Geometry: see drawing. Coordinates: mm, zero at the bounding-box minimum. Coordinates: 2 decimals unless noted, no trailing zeros. Loops run counter-clockwise (first coordinate to the right, second up) from the corner with the lowest first, then second, coordinate; pieces in that order, holes last. Notation, with made-up numbers: (75, 55.5) - (120, 55.5) arc R25 ccw to (120, 70.5) - close; hole circle Ø8 at (-20.75, -26). An arc over 180 degrees is marked (long way). Use one line per item in the form item = value.
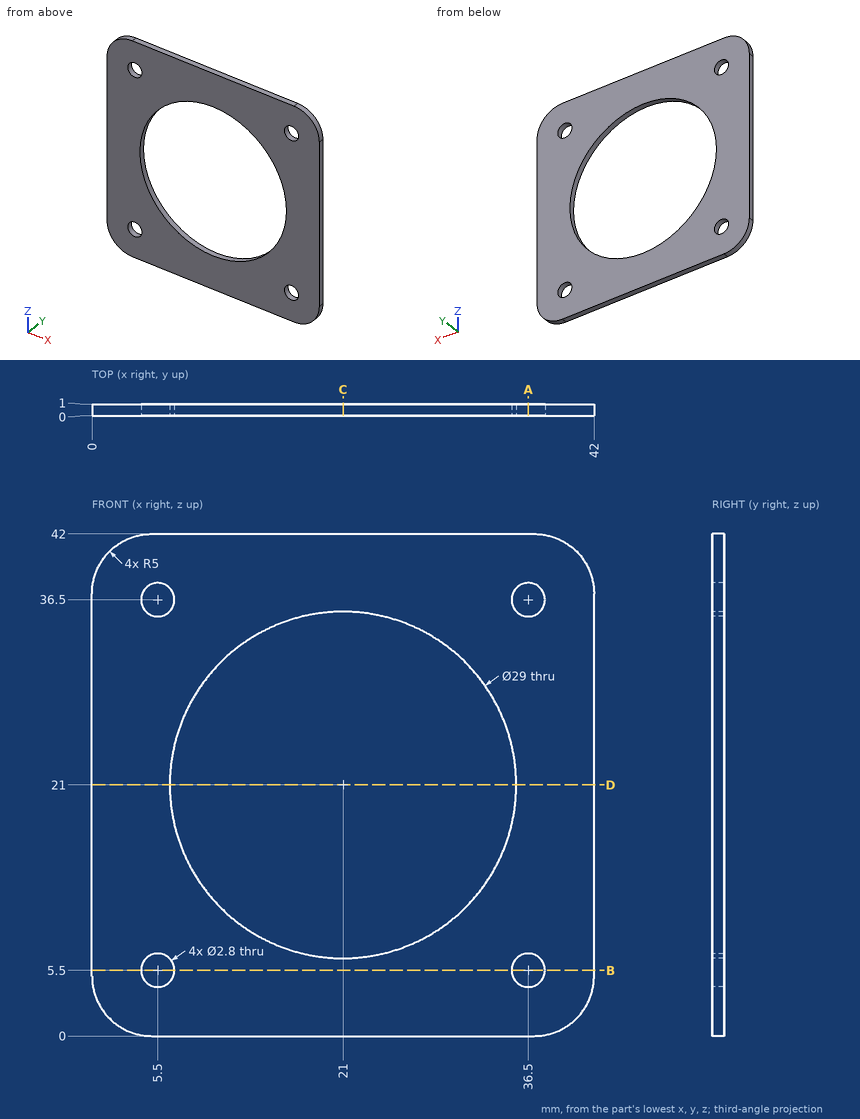
Q1. Cut plane B-B, the plane z = 5.5. Return loops of the section in (x, y).
Check values:
outline = (0, 0) - (4.1, 0) - (4.1, 1) - (0, 1) - close; (6.9, 0) - (35.1, 0) - (35.1, 1) - (6.9, 1) - close; (37.9, 0) - (42, 0) - (42, 1) - (37.9, 1) - close
Q2. First-contact query: P1, Ø3.5, axis at x = 5.5, z = 5.5, coming from the +Y side. Flat tip, straight axial feed; report the tip coordinate or a pass-through.
Check values:
P1 = 1
Q3. Cut plane A-A, the plane x = 36.5. Return loops of the section in (y, z), then the cut area to 3 significant figures.
Check values:
outline = (0, 0) - (1, 0) - (1, 4.1) - (0, 4.1) - close; (0, 6.9) - (1, 6.9) - (1, 35.1) - (0, 35.1) - close; (0, 37.9) - (1, 37.9) - (1, 42) - (0, 42) - close
area = 36.4 mm²
Q4. Cut plane D-D, the plane z = 21. Return loops of the section in (x, y), then the cut area to 3 significant figures.
Check values:
outline = (0, 0) - (6.5, 0) - (6.5, 1) - (0, 1) - close; (35.5, 0) - (42, 0) - (42, 1) - (35.5, 1) - close
area = 13.0 mm²
Q5. Ray query, line 1 along Z through (x, y) = (5.5, 0.6); line 2 along X through (y, z) = (0.15, 20.5). Return the intervals inside material, ascending. Write a range as [from, to].
Check values:
line_1 = [0, 4.1], [6.9, 35.1], [37.9, 42]
line_2 = [0, 6.51], [35.49, 42]
Q6. Cut plane C-C, the plane x = 21. Return loops of the section in (y, z).
Check values:
outline = (0, 0) - (1, 0) - (1, 6.5) - (0, 6.5) - close; (0, 35.5) - (1, 35.5) - (1, 42) - (0, 42) - close
